Could you check a few things on this model? Use its own coordinates, in mm. A direction names the side the tool comes from. Coordinates: 2 decimals unless noted, no trailing zeros. Write each loop counter-clockwise with the first axis right and the second up, starting at its lowest first coordinate (ties: lowest second). Pieces come first, ordered by that corner, then holes. Notation, with made-up numbers: (34.25, 59) - (91.25, 59) arc R22 ccw to (91.25, 88) - close; hole circle Ø2 at (77, 68). An arc over 180 degrees is marked (long way). Answer as a JSON object with one key per item and string values. Group by question number.
1) If we section it at C-C (y = 1.5): Write out the boundary of the cut face in (x, z) (3 decimals).
2) If we section it at A-A (x = 76): Write out the boundary of the cut face in (y, z) (1 decimal), plus the area to 3 significant figures.
3) If we section it at B-B (z = 28.5): Write out the boundary of the cut face in (x, y) (3 decimals).
4) We'd pull the mould along X, two halves only. Please class faces 4 (the cylindrical face through (53.45, 4.832, 125.097)), 5 (the flat face through (62.706, 5, 123)), 6 (the flat face through (64.294, 5, 124)), 7 (the flat face through (0, 5, 59)): released by +X, released by -X, zero draft, split by the parting line, or undercut.
5) On a 3-axis mill with a long thin cutter (end or side, diameter ignored), from which of +Z, -Z, +X, -X, +Y, -Y can I reach the whole of each face in a straight line? I mean faces 1 (the flat face through (44.45, 5, 124)), 2 (the cylindrical face through (62.355, 4.829, 52.073)), 3 (the flat face through (82.55, 5, 124)). Say none if no direction works.
6) Please list where these lines run through material, in increasing order: line 1 along X through (y, z) = (6.25, 94); line 2 along Z through (x, y) = (71, 5.75) (3 decimals); line 3 along X through (y, z) = (3.5, 119).
7) If we section it at D-D (z = 99.5): Write out the boundary of the cut face in (x, y) (3 decimals).
8) Will these pins go through, and if not, where does the flat tip stop? pin 1 Ø3 at (y, z) = (4.76, 126.68) entering from +X; pin 2 Ø3 at (y, z) = (4, 120) entering from -X; pin 3 Ø5 at (x, y) = (113.5, 5) entering from -Z.
```python
from build123d import *

# Parameters (mm, degrees)
SKETCH1_W           = 127
SKETCH1_H           = 131.445
BOSS_EXTRUDE1_DEPTH = 9.525
SKETCH2_W           = 44.45
SKETCH2_H           = 15.875
CUT_EXTRUDE1_DEPTH  = 10.525
CUT_EXTRUDE2_DEPTH  = 10.525
CUT_EXTRUDE3_DEPTH  = 10.525
SKETCH6_R           = 1.5875
CUT_EXTRUDE4_DEPTH  = 83.55


with BuildPart() as part:
    # Sketch1 → Boss-Extrude1 (new body)
    with BuildSketch(Plane(origin=(0, 0, 0), x_dir=(1, 0, 0), z_dir=(0, 1, 0))):
        with Locations((63.5, -65.7225)):
            Rectangle(SKETCH1_W, SKETCH1_H)
    extrude(amount=BOSS_EXTRUDE1_DEPTH)

    # Sketch2 → Cut-Extrude1 (cut, through all)
    with BuildSketch(Plane(origin=(0, 9.525, 0), x_dir=(1, 0, 0), z_dir=(0, 1, 0))):
        with Locations((22.225, -123.5075)):
            Rectangle(SKETCH2_W, SKETCH2_H)
        with Locations((104.775, -123.5075)):
            Rectangle(SKETCH2_W, SKETCH2_H)
    extrude(amount=-CUT_EXTRUDE1_DEPTH, mode=Mode.SUBTRACT)

    # Sketch3 → Cut-Extrude2 (cut, through all)
    with BuildSketch(Plane(origin=(0, 9.525, 0), x_dir=(1, 0, 0), z_dir=(0, 1, 0))):
        with BuildLine():
            Line((63.5, -131.445), (64.29375, -131.445))
            Line((64.29375, -131.445), (64.29375, -115.57))
            Line((64.29375, -115.57), (64.29375, -115.55496146))
            ThreePointArc((64.29375, -115.55496146), (63.5, -73.66), (62.70625, -115.55496146))
            Line((62.70625, -115.55496146), (62.70625, -115.57))
            Line((62.70625, -115.57), (62.70625, -131.445))
            Line((62.70625, -131.445), (63.5, -131.445))
        make_face()
    extrude(amount=-CUT_EXTRUDE2_DEPTH, mode=Mode.SUBTRACT)

    # Sketch5 → Cut-Extrude3 (cut, through all)
    with BuildSketch(Plane(origin=(0, 9.525, 0), x_dir=(1, 0, 0), z_dir=(0, 1, 0))):
        with BuildLine():
            ThreePointArc((11.41476, 0), (63.5, -52.08524), (115.58524, 0))
            Line((115.58524, 0), (11.41476, 0))
        make_face()
        with BuildLine():
            Line((11.41476, 0), (115.58524, 0))
            ThreePointArc((115.58524, 0), (63.5, 52.08524), (11.41476, 0))
        make_face()
    extrude(amount=-CUT_EXTRUDE3_DEPTH, mode=Mode.SUBTRACT)

    # Sketch6 → Cut-Extrude4 (cut, through all)
    with BuildSketch(Plane.ZY.offset(-44.45)):
        with Locations((120.3325, 4.7625)):
            Circle(SKETCH6_R)
        with Locations((126.6825, 4.7625)):
            Circle(SKETCH6_R)
    extrude(amount=-CUT_EXTRUDE4_DEPTH, mode=Mode.SUBTRACT)


solid = part.part
```
Here are the results:
{
 "1": {"outline": "(0, 0) - (11.415, 0) arc R52.085 cw to (115.585, 0) - (127, 0) - (127, 115.57) - (82.55, 115.57) - (82.55, 131.445) - (64.294, 131.445) - (64.294, 115.555) arc R20.955 cw (long way) to (62.706, 115.555) - (62.706, 131.445) - (44.45, 131.445) - (44.45, 115.57) - (0, 115.57) - close"},
 "2": {"outline": "(0, 50.6) - (9.5, 50.6) - (9.5, 77.8) - (0, 77.8) - close; (0, 111.4) - (9.5, 111.4) - (9.5, 131.4) - (0, 131.4) - close; hole circle Ø3.2 at (4.8, 120.3); hole circle Ø3.2 at (4.8, 126.7)", "area": "434 mm²"},
 "3": {"outline": "(0, 0) - (19.904, 0) - (19.904, 9.525) - (0, 9.525) - close; (107.096, 0) - (127, 0) - (127, 9.525) - (107.096, 9.525) - close"},
 "4": {"face 4": "zero draft", "face 5": "undercut", "face 6": "undercut", "face 7": "released by -X"},
 "5": {"face 1": "+Z, -X, +Y, -Y", "face 2": "-Z, +Y, -Y", "face 3": "+Z, +X, +Y, -Y"},
 "6": {"line 1": "x = 0 to 42.55, 84.45 to 127", "line 2": "z = 51.542 to 75.048, 114.182 to 119.09, 121.575 to 125.44, 127.925 to 131.445", "line 3": "x = 44.45 to 62.71, 64.29 to 82.55"},
 "7": {"outline": "(0, 0) - (43.122, 0) - (43.122, 9.525) - (0, 9.525) - close; (83.878, 0) - (127, 0) - (127, 9.525) - (83.878, 9.525) - close"},
 "8": {"pin 1": "passes through", "pin 2": "stops at x = 44.45", "pin 3": "stops at z = 0"}
}
